```python
from build123d import *

# Parameters (mm, degrees)
SKIZZE1_R                            = 4
AUFSATZ_LINEAR_AUSTRAGEN1_DEPTH      = 65
SKIZZE2_R                            = 4.25
AUFSATZ_LINEAR_AUSTRAGEN2_DEPTH      = 20
SKIZZE3_R                            = 2
SCHNITT_LINEAR_AUSTRAGEN1_DEPTH      = 5.25
SCHNITT_LINEAR_AUSTRAGEN1_DEPTH_BACK = 5.25
FASE1_SIZE                           = 1
SKIZZE4_R                            = 4
SKIZZE4_R_2                          = 3.5
SCHNITT_LINEAR_AUSTRAGEN2_DEPTH      = 22


with BuildPart() as part:
    # Skizze1 → Aufsatz-Linear austragen1 (new body)
    with BuildSketch(Plane.XY):
        Circle(SKIZZE1_R)
    extrude(amount=AUFSATZ_LINEAR_AUSTRAGEN1_DEPTH)

    # Skizze2 → Aufsatz-Linear austragen2 (add)
    with BuildSketch(Plane(origin=(0, 0, 0), x_dir=(-1, 0, 0), z_dir=(0, 0, -1))):
        Circle(SKIZZE2_R)
    extrude(amount=-AUFSATZ_LINEAR_AUSTRAGEN2_DEPTH)

    # Skizze3 → Schnitt-Linear austragen1 (cut, two sides)
    with BuildSketch(Plane(origin=(0, 0, 0), x_dir=(0, 0, -1), z_dir=(1, 0, 0))) as schnitt_linear_austragen1_sk:
        with Locations((-12, 0)):
            Circle(SKIZZE3_R)
    extrude(amount=SCHNITT_LINEAR_AUSTRAGEN1_DEPTH, mode=Mode.SUBTRACT)
    extrude(schnitt_linear_austragen1_sk.sketch, amount=-SCHNITT_LINEAR_AUSTRAGEN1_DEPTH_BACK, mode=Mode.SUBTRACT)

    # Fase1
    fase1_edges = [part.edges().sort_by_distance(p)[0] for p in [
        (4.25, 0, 0),
    ]]
    chamfer(fase1_edges, length=FASE1_SIZE)

    # Skizze4 → Schnitt-Linear austragen2 (cut)
    with BuildSketch(Plane.XY.offset(65)):
        Circle(SKIZZE4_R)
        Circle(SKIZZE4_R_2, mode=Mode.SUBTRACT)
    extrude(amount=-SCHNITT_LINEAR_AUSTRAGEN2_DEPTH, mode=Mode.SUBTRACT)


solid = part.part
```
The listing builds one solid part. Answer for the finished solid, in the listing's coordinates (mm). A direction names the side the tool comes from. Round coordinates to 2 decimals unless told otherwise and drop trailing zeros. Order: outer loops, then holes, each group sorted by start corner. A loop starts at its lowest first (then second) coordinate and runs counter-clockwise, first axis right, second up. Notation, with made-up numbers: (37.25, 19.25) - (87.25, 19.25) arc R17 ccw to (87.25, 26.25) - close; hole circle Ø11 at (-24, 36.5). An arc over 180 degrees is marked (long way). Put each result on its own line as item: value. Start each with the question number.
(1) For faces 4 (the cylindrical face through (-0.867, -3.905, 31.339)), 5 (the cylindrical face through (-3.926, -1.628, 10.367)), determine the directions among +Z, -Z, +X, -X, +Y, -Y from which every point of the face is accessible in a straight line to the end or side of a thin tool.
(2) Find section D-D (z = 44). Give the vertices of the cut face in (x, y).
(3) Determine the mould class of faces 1 (the flat face through (0, 0, 0)), 2 (the cylindrical face through (3.233, -1.341, 54.154)), 3 (the cylindrical face through (0.059, 0.601, 10.092)) for opening direction Z: released by +Z, released by -Z, zero draft, split by the parting line, or undercut.
(4) Straight lines are drawn through the part: probe 1 along Z at (x, y) = (-2, 0); probe 2 along Z at (x, y) = (-1, -0.5); probe 3 along X at (y, z) = (0.25, 53). For each, find the intervals that lie inside material, in ascending order. Write a range as from..to.
(5) Find section C-C (z = 12). Give the vertices of the cut face in (x, y), plus the area to 3 significant figures.
(6) Find section B-B (x = 0). Give the vertices of the cut face in (y, z), plus the area to 3 significant figures.
(7) Given P1, Ø2, axis at y = -3, z = 45, coming from the -X side; P2, Ø4, axis at x = 1.5, z = 56, coming from the +Y side; P3, Ø3, axis at x = 3, z = 10, coming from the +Y side; P4, Ø5, axis at y = 0, z = 12, coming from the -X side, each flat-ended and moving along its own axis, determine where each tip first touches the part or whether it passes through.
(8) Find section A-A (y = 0). Give the vertices of the cut face in (x, z).
Reply:
1. face 4: +Z
1. face 5: +Z, -Z
2. outline: circle Ø7 at (0, 0)
3. face 1: released by -Z
3. face 2: zero draft
3. face 3: undercut
4. probe 1: 0..10, 14..65
4. probe 2: 0..10.06, 13.94..65
4. probe 3: -3.49..3.49
5. outline: (-3.75, -2) arc R4.25 ccw to (3.75, -2) - close; (-3.75, 2) - (3.75, 2) arc R4.25 ccw to start
5. area: 24.0 mm^2
6. outline: (-4.25, 1) - (-3.25, 0) - (3.25, 0) - (4.25, 1) - (4.25, 20) - (4, 20) - (4, 43) - (3.5, 43) - (3.5, 65) - (-3.5, 65) - (-3.5, 43) - (-4, 43) - (-4, 20) - (-4.25, 20) - close; hole circle Ø4 at (0, 12)
6. area: 494 mm^2
7. P1: x = -2.87
7. P2: y = 3.5
7. P3: y = 3.98
7. P4: x = -4.25
8. outline: (-4.25, 1) - (-3.25, 0) - (3.25, 0) - (4.25, 1) - (4.25, 10) - (-4.25, 10) - close; (-4.25, 14) - (4.25, 14) - (4.25, 20) - (4, 20) - (4, 43) - (3.5, 43) - (3.5, 65) - (-3.5, 65) - (-3.5, 43) - (-4, 43) - (-4, 20) - (-4.25, 20) - close
